Can you work these out from the model? Positions are in its coordinate system, mm. A direction names the side the tool comes from. Give positions to 0.01 mm unless a question says otherwise; leave off trailing zeros. Write each loop counter-clockwise with the first axis right and the second up, starting at its lowest first coordinate (ties: lowest second). Pieces come first, ordered by that corner, then holes.
1. On a 3-axis mill with a long thin cutter (end or side, diameter ignored), from which of +Z, -Z, +X, -X, +Y, -Y can I reach the whole of each face in a straight line? I mean faces 1 (the flat face through (0, 18, 180)), 2 (the flat face through (0.3, -4.2, -6.35)). Say none if no direction works.
2. Suppose I cut it at C-C (y = 33). Please give me the cut outline in (x, z).
3. If I drill on probe 1 along Y at (x, z) = (0.45, 139.7); probe 2 along Z at (x, y) = (1.1, 6.35); probe 3 along X at (y, z) = (1.5, 81.5), over which ranges is the centre line in solid material (lowest first)?
4. I'm going to push flat-ended pins straight in: pin 1 (2 mm diameter, centred on x = -3, y = -14, fed in from +Z); pin 2 (12 mm diameter, centred on x = -8.5, z = 55, fed in from +Y) (3 decimals); pin 3 (4 mm diameter, centred on y = 0, z = 0, fed in from -X); pin 4 (5 mm diameter, centred on x = -5.5, z = 214, fed in from -Y). Where does each tip first touch, or does it pass through?
Autodesk Inventor part; units mm, degrees
ref_plane "YZ Plane" through (0, 0, 0) normal (1, 0, 0) x (0, 1, 0)
ref_plane "XZ Plane" through (0, 0, 0) normal (0, 1, 0) x (-1, 0, 0)
ref_plane "XY Plane" through (0, 0, 0) normal (0, 0, 1) x (1, 0, 0)
sketch "main" plane through (0, 0, 0) normal (0, 0, 1) x (1, 0, 0)
  circle A0 centre (51.9329, 240.4167) radius 2.1844
  line L0 (60.6642, 253.1167) -> (43.2017, 253.1167)
  arc A1 (32.8829, 253.1167) -> (7.4829, 227.7167) centre (32.8829, 227.7167) ccw
  line L1 (39.2329, 253.1167) -> (32.8829, 253.1167)
  line L2 (39.2329, 249.9417) -> (39.2329, 253.1167)
  line L3 (39.2329, 253.1167) -> (42.4079, 253.1167)
  line L4 (42.4079, 253.1167) -> (43.2017, 253.1167)
  arc A2 (65.1185, 250.5268) -> (61.9979, 253.1167) centre (61.9979, 249.9417) ccw
  line L5 (61.9979, 253.1167) -> (60.6642, 253.1167)
  line L6 (42.4079, -115.1833) -> (62.5393, -115.1833)
  arc A3 (7.4829, -102.4833) -> (20.1829, -115.1833) centre (20.1829, -102.4833) ccw
  line L7 (20.1829, -115.1833) -> (42.4079, -115.1833)
  arc A4 (62.5393, -115.1833) -> (65.4576, -113.259) centre (62.5393, -112.0083) ccw
  line L8 (39.2329, 249.9417) -> (39.2329, -115.1833)
  line L9 (102.4762, -26.8823) -> (65.4576, -113.259)
  line L10 (102.7329, -25.6316) -> (102.7329, 49.6216)
  line L11 (102.6786, 50.2068) -> (65.1185, 250.5268)
  line L12 (7.4829, 227.7167) -> (7.4829, -102.4833)
  arc A5 (102.7329, 49.6216) -> (102.6786, 50.2068) centre (99.5579, 49.6216) ccw
  circle A6 centre (96.3829, 30.8667) radius 2.1844
  circle A7 centre (96.3829, -7.2333) radius 2.1844
  arc A8 (102.4762, -26.8823) -> (102.7329, -25.6316) centre (99.5579, -25.6316) ccw
  circle A9 centre (45.5829, -108.8333) radius 2.1844
  point P0 (57.0821, 72.2396)
  point P1 (7.4829, 253.1167)
  point P2 (64.6329, -115.1833)
  point P3 (102.7329, -26.2833)
  dimension "d0" = 25.4
  dimension "d1" = 3.175
  dimension "d2" = 3.175
  dimension "d3" = 3.175
  dimension "d4" = 31.75
  dimension "d5" = 90
  dimension "d6" = 25.4
  dimension "d7" = 12.7
sketch "Sketch1" plane through (0, 0, 0) normal (1, 0, 0) x (0, 1, 0)
  circle A0 centre (6.35, 349.25) radius 2.1844
  line L0 (15.0812, 361.95) -> (-2.3813, 361.95)
  arc A1 (-12.7, 361.95) -> (-38.1, 336.55) centre (-12.7, 336.55) ccw
  line L1 (-6.35, 361.95) -> (-12.7, 361.95)
  line L2 (-6.35, 358.775) -> (-6.35, 361.95)
  line L3 (-6.35, 361.95) -> (-3.175, 361.95)
  line L4 (-3.175, 361.95) -> (-2.3813, 361.95)
  arc A2 (19.5356, 359.3601) -> (16.415, 361.95) centre (16.415, 358.775) ccw
  line L5 (16.415, 361.95) -> (15.0812, 361.95)
  line L6 (-3.175, -6.35) -> (16.9564, -6.35)
  arc A3 (-38.1, 6.35) -> (-25.4, -6.35) centre (-25.4, 6.35) ccw
  line L7 (-25.4, -6.35) -> (-3.175, -6.35)
  arc A4 (16.9564, -6.35) -> (19.8747, -4.4257) centre (16.9564, -3.175) ccw
  line L8 (-6.35, 358.775) -> (-6.35, -6.35)
  line L9 (56.8933, 81.951) -> (19.8747, -4.4257)
  line L10 (57.15, 83.2017) -> (57.15, 158.4549)
  line L11 (57.0956, 159.04) -> (19.5356, 359.3601)
  line L12 (-38.1, 336.55) -> (-38.1, 6.35)
  arc A5 (57.15, 158.4549) -> (57.0956, 159.04) centre (53.975, 158.4549) ccw
  circle A6 centre (50.8, 139.7) radius 2.1844
  circle A7 centre (50.8, 101.6) radius 2.1844
  arc A8 (56.8933, 81.951) -> (57.15, 83.2017) centre (53.975, 83.2017) ccw
  circle A9 centre (0, 0) radius 2.1844
extrude "Extrusion1" add sketch "Sketch1" along normal blind 1.5875
bend part "Bend Part1" radius 3.175 angle 40 line through (0, -6.35, 358.775) along (0, 0, -1) centre toward (-1, 0, 0) moving side (0, -1, 0) both sides no
properties part number "side_panel_mirrored" material "Acetal Resin, White"
Checks:
1. face 1: +Z, -Z, -X, +Y
1. face 2: -Z, +X, -X, +Y, -Y
2. outline: (0, 26.2) - (1.59, 26.2) - (1.59, 287.55) - (0, 287.55) - close
3. probe 1: y = -9.44 to 48.62, 52.98 to 57.15
3. probe 2: z = -6.35 to 347.07, 351.43 to 361.95
3. probe 3: x = 0 to 1.59
4. pin 1: stops at z = 361.94
4. pin 2: stops at y = -10.485
4. pin 3: passes through
4. pin 4: stops at y = -19.51
